from build123d import *

# Parameters (mm, degrees)
BOSS_EXTRUDE1_DEPTH  = 20
FILLET1_R            = 50
CUT_EXTRUDE3_DEPTH   = 20
FILLET3_R            = 15
FILLET1_OF_MIRROR2_R = 50
FILLET3_OF_MIRROR2_R = 15


with BuildPart() as part:
    # Sketch1 → Boss-Extrude1 (new body)
    with BuildSketch(Plane(origin=(0, 0, 0), x_dir=(1, 0, 0), z_dir=(0, 1, 0))):
        Polygon((-75, 35), (-75, 0), (0, 0), (0, 280), (-145, 280), (-6.056000119, 92.850884872), align=None)
    boss_extrude1 = extrude(amount=BOSS_EXTRUDE1_DEPTH)

    # Fillet1
    fillet1_edges = [part.edges().sort_by_distance(p)[0] for p in [
        (-6.056000119, 10, -92.850884872),
    ]]
    fillet(fillet1_edges, radius=FILLET1_R)

    # Sketch5 → Cut-Extrude3 (cut)
    with BuildSketch(Plane(origin=(0, 20, 0), x_dir=(1, 0, 0), z_dir=(0, 1, 0))):
        with BuildLine():
            Line((0, 190), (0, 280))
            Line((0, 280), (-90, 280))
            ThreePointArc((-90, 280), (-63.639610307, 216.360389693), (0, 190))
        make_face()
        with BuildLine():
            Line((-145, 280), (-93.476414041, 210.60086417))
            ThreePointArc((-93.476414041, 210.60086417), (-110.536849713, 243.452976984), (-116.421991204, 280))
            Line((-116.421991204, 280), (-145, 280))
        make_face()
    cut_extrude3 = extrude(amount=-CUT_EXTRUDE3_DEPTH, mode=Mode.SUBTRACT)

    # Fillet3
    fillet3_edges = [part.edges().sort_by_distance(p)[0] for p in [
        (-116.421991204, 10, -280),
    ]]
    fillet(fillet3_edges, radius=FILLET3_R)

    # Mirror2: Boss-Extrude1, Cut-Extrude3 across plane
    add(boss_extrude1.mirror(Plane(origin=(0, 20, 0), x_dir=(0, 0, 1), z_dir=(-1, 0, 0))))
    add(cut_extrude3.mirror(Plane(origin=(0, 20, 0), x_dir=(0, 0, 1), z_dir=(-1, 0, 0))), mode=Mode.SUBTRACT)

    # Fillet1 of Mirror2
    fillet1_of_mirror2_edges = [part.edges().sort_by_distance(p)[0] for p in [
        (6.056000119, 10, -92.850884872),
    ]]
    fillet(fillet1_of_mirror2_edges, radius=FILLET1_OF_MIRROR2_R)

    # Fillet3 of Mirror2
    fillet3_of_mirror2_edges = [part.edges().sort_by_distance(p)[0] for p in [
        (116.421991204, 10, -280),
    ]]
    fillet(fillet3_of_mirror2_edges, radius=FILLET3_OF_MIRROR2_R)


solid = part.part
Design review of the part built by this model. Coordinates are the model's own, in mm. A direction names the side the tool comes from. Coordinates: 2 decimals unless noted, no trailing zeros. Loops run counter-clockwise (first coordinate to the right, second up) from the corner with the lowest first, then second, coordinate; pieces in that order, holes last. Notation, with made-up numbers: (45, 57.5) -> (73, 57.5) arc R26 cw to (73, 81.5) -> close; hole circle Ø9 at (-10.75, -3). An arc over 180 degrees is marked (long way). Use a Markdown table: item, result. Add a question column.
Item 1: Clearance check with flat-ended pins moving along their axes: P1, Ø10, axis at x = -24, y = 3, coming from the -Z side; P2, Ø6, axis at y = 9.5, z = -15.5, coming from the -X side; P3, Ø4, axis at x = -25, y = 9, coming from the -Z side; P4, Ø6, axis at x = -28.5, z = -96, coming from the -Y side. State where each tip first meets the part, or that it passes through.
Item 2: The part is to be moulded in two halves that separate along Z. For faces 1 (the cylindrical face through (-107.37, 10.14, -234.99)), 2 (the flat face through (95, 10, -280)), 3 (the flat face through (-58.34, 9.86, -48.98)), say which applies: +Z half, -Z half, draft (parallel to the pull), parting line (faces both ways), or undercut.
Item 3: Wall thickness on L1, parallel to Z at x = -51, y = 9; L2, parallel to Z at x = 64.5, y = 17; L3, parallel to X at y = 16.25, z = -101.5: over which ranges is each line inside the solid? List them lowest first. Write a range as from..to.
Item 4: We need section A-A, the plane z = -255. Write out the cut boundary in (x, y), and give its area (3 significant figures).
Item 5: We need section B-B, the plane x = -62. Write out the cut boundary in (y, z), and give its area (3 significant figures).
Item 6: Machinability: for faces 4 (the flat face through (75, 10, -18)), 5 (the flat face through (2, 0, -142)), 6 (the flat face through (58.34, 9.86, -48.98)), 7 (the flat face through (-75, 10, -18)), 8 (the flat face through (-64.223, 9.86, -171.198)), which of the approach directions +Z, -Z, +X, -X, +Y, -Y give a long, thin tool a straight path to every point of the face, cutting with its end or side? Answer none if there is none.
Item 7: We need section C-C, the plane y = 14.5. Write out the cut boundary in (x, z).
Item 8: We need section D-D, the plane x = -13. Write out the cut boundary in (y, z).
Numbers:
| question | item | result |
|---|---|---|
| 1 | P1 | stops at z = -194.8 |
| 1 | P2 | stops at x = -75 |
| 1 | P3 | stops at z = -194.15 |
| 1 | P4 | passes through |
| 2 | face 1 | +Z half |
| 2 | face 2 | -Z half |
| 2 | face 3 | undercut |
| 3 | L1 | z = -205.84..-153.39, -55.14..0 |
| 3 | L2 | z = -217.23..-171.57, -43.81..0 |
| 3 | L3 | x = -24.29..24.29 |
| 4 | outline | (-113.71, 0) -> (-86.46, 0) -> (-86.46, 20) -> (-113.71, 20) -> close; (86.46, 0) -> (113.71, 0) -> (113.71, 20) -> (86.46, 20) -> close |
| 4 | area | 1,090 mm^2 |
| 5 | outline | (0, -214.76) -> (20, -214.76) -> (20, -168.2) -> (0, -168.2) -> close; (0, -45.91) -> (20, -45.91) -> (20, 0) -> (0, 0) -> close |
| 5 | area | 1,850 mm^2 |
| 6 | face 4 | +Z, +X, +Y, -Y |
| 6 | face 5 | +Z, -Z, +X, -X, -Y |
| 6 | face 6 | +X, +Y, -Y |
| 6 | face 7 | +Z, -X, +Y, -Y |
| 6 | face 8 | -X, +Y, -Y |
| 7 | outline | (-115.14, -262.78) arc R15 ccw to (-100.31, -280) -> (-90, -280) arc R90 cw to (90, -280) -> (100.31, -280) arc R15 ccw to (115.14, -262.78) arc R116.42 ccw to (93.48, -210.6) -> (34.14, -130.68) arc R50 cw to (42.14, -62.57) -> (75, -35) -> (75, 0) -> (-75, 0) -> (-75, -35) -> (-42.14, -62.57) arc R50 cw to (-34.14, -130.68) -> (-93.48, -210.6) arc R116.42 ccw to start |
| 8 | outline | (0, -190.94) -> (20, -190.94) -> (20, 0) -> (0, 0) -> close |
